Geometry check sheet. Reference: the model listing, model coordinates, mm. A direction names the side the tool comes from. Give positions to 0.01 mm unless a question says otherwise; leave off trailing zeros. Write each loop counter-clockwise with the first axis right and the second up, starting at its lowest first coordinate (ties: lowest second). Pieces come first, ordered by that corner, then holes.
(1) Cross-section at C-C (y = -8.5). Record the boundary of the cut face in (x, z), and give its area (3 significant figures).
(2) Mould release check, pull along X, two halves, no side actions. Record for faces 1 (the flat face through (22, -6, 1.5)), 2 (the cylindrical face through (-7.8, -7.03, 3.94)), 3 (the cylindrical face through (24.76, -3.65, 0.74)), 4 (the flat face through (10, 1, 0)): +X half, -X half, draft (parallel to the pull), parting line (faces both ways), or undercut.
(3) Tool access check on faces 5 (the flat face through (30.5, 5, 4)), 6 (the flat face through (10, 10, 4)), 7 (the cylindrical face through (-0.92, 7.04, 4.71)). Record the directions out of +Z, -Z, +X, -X, +Y, -Y that give a thin tool (end or side, any length) a straight path to the whole face; none if there is none.
(4) Thickness scan on line 1 along Y through (x, z) = (20, 4.65); line 2 along X through (y, z) = (0.75, 2.25); line 3 along X through (y, z) = (-6.5, 6.25). Record the ranges inside material, lowest first.
(5) Cross-section at A-A (z = 5.5). Record the boundary of the cut face in (x, y).
(6) Depth check by flat-ended pin: P1, Ø5, axis at x = 14, y = 2.5, coming from the +Z side; P2, Ø0.5, axis at y = 11, z = 2, coming from the +X side; P3, Ø8.5, axis at x = 0, y = 0, coming from the +Z side; P4, Ø2.5, axis at x = 9.5, z = 3, coming from the +Y side. Enter the tip coordinate at first touch or a pass-through.
(7) Cross-section at B-B (y = -2). Count the separate pieces of the cut face and the enclosed holes in it, and give its area (3 significant figures).
```python
from build123d import *

# Parameters (mm, degrees)
SKETCH1_R               = 7.1
BOSS_EXTRUDE1_DEPTH     = 8
SKETCH2_R               = 7.1
SKETCH2_R_2             = 6
BOSS_EXTRUDE2_DEPTH     = 1.5
SKETCH3_W               = 10
SKETCH3_H               = 10
CUT_EXTRUDE1_DEPTH      = 31.5
CUT_EXTRUDE1_DEPTH_BACK = 10
FILLET4_R               = 1
CHAMFER1_SIZE           = 0.4


with BuildPart() as part:
    # Sketch1 → Boss-Extrude1 (new body)
    with BuildSketch(Plane.XY):
        with BuildLine():
            Line((-12, 2), (-10.345741649, 1.793217706))
            ThreePointArc((-10.345741649, 1.793217706), (-8.033641326, -6.760961991), (0, -10.5))
            Line((0, -10.5), (20, -10.5))
            ThreePointArc((20, -10.5), (27.424621202, -7.424621202), (30.5, 0))
            Line((30.5, 0), (30.5, 10.5))
            Line((30.5, 10.5), (0, 10.5))
            Line((0, 10.5), (-12, 12))
            Line((-12, 12), (-12, 2))
        make_face()
        with Locations((20, 0)):
            Circle(SKETCH1_R, mode=Mode.SUBTRACT)
        Circle(SKETCH1_R, mode=Mode.SUBTRACT)
    extrude(amount=BOSS_EXTRUDE1_DEPTH)

    # Sketch2 → Boss-Extrude2 (add)
    with BuildSketch(Plane(origin=(0, 0, 0), x_dir=(-1, 0, 0), z_dir=(0, 0, -1))):
        with Locations((-20, 0)):
            Circle(SKETCH2_R)
        with Locations((-20, 0)):
            Circle(SKETCH2_R_2, mode=Mode.SUBTRACT)
        Circle(SKETCH2_R)
        Circle(SKETCH2_R_2, mode=Mode.SUBTRACT)
    extrude(amount=-BOSS_EXTRUDE2_DEPTH)

    # Sketch3 → Cut-Extrude1 (cut, two sides)
    with BuildSketch(Plane(origin=(0, 0, 0), x_dir=(0, 0, -1), z_dir=(1, 0, 0))) as cut_extrude1_sk:
        with Locations((-4, 15)):
            Rectangle(SKETCH3_W, SKETCH3_H)
    extrude(amount=CUT_EXTRUDE1_DEPTH, mode=Mode.SUBTRACT)
    extrude(cut_extrude1_sk.sketch, amount=-CUT_EXTRUDE1_DEPTH_BACK, mode=Mode.SUBTRACT)

    # Fillet4
    fillet4_edges = [part.edges().sort_by_distance(p)[0] for p in [
        (-10.345741649, 1.793217706, 4),
    ]]
    fillet(fillet4_edges, radius=FILLET4_R)

    # Chamfer1
    chamfer1_edges = [part.edges().sort_by_distance(p)[0] for p in [
        (12.9, 0, 1.5),
        (-7.1, 0, 1.5),
        (12.9, 0, 8),
        (-7.1, 0, 8),
    ]]
    chamfer(chamfer1_edges, length=CHAMFER1_SIZE)


solid = part.part
```
Reply:
1. outline: (-6.16, 0) - (26.16, 0) - (26.16, 8) - (-6.16, 8) - close
1. area: 259 mm2
2. face 1: undercut
2. face 2: -X half
2. face 3: undercut
2. face 4: draft
3. face 5: +Z, -Z, +X, +Y, -Y
3. face 6: +Z, -Z, +X, +Y
3. face 7: +Z
4. line 1: y = -10.5 to -7.1, 7.1 to 10
4. line 2: x = -10.47 to -7.06, 7.06 to 12.94, 27.06 to 30.5
4. line 3: x = -8.25 to -2.86, 2.86 to 17.14, 22.86 to 28.25
5. outline: (-12, 2) - (-11.34, 1.92) arc R1 cw to (-10.47, 0.84) arc R10.5 ccw to (0, -10.5) - (20, -10.5) arc R10.5 ccw to (30.5, 0) - (30.5, 10) - (-10, 10) - (-10, 11.75) - (-12, 12) - close; hole circle Ø14.2 at (0, 0); hole circle Ø14.2 at (20, 0)
6. P1: stops at z = 8
6. P2: stops at x = -10
6. P3: passes through
6. P4: stops at y = 10
7. separate pieces: 3
7. enclosed holes: 0
7. area: 114 mm2
